```python
from build123d import *

# Parameters (mm, degrees)
SKETCH1_W                                        = 254
SKETCH1_H                                        = 25.4
BOSS_EXTRUDE1_DEPTH                              = 12.7
SKETCH2_R                                        = 5.08
F_1_2_20_THREAD_THRU_DEPTH                       = 256.582569828
SKETCH4_R                                        = 4.1021
CUT_EXTRUDE4_DEPTH                               = 256.582569828
CSK_FOR_1_4_FLAT_HEAD_MACHINE_SCREW1_D           = 6.5278
CSK_FOR_1_4_FLAT_HEAD_MACHINE_SCREW1_CSINK_D     = 12.8778
CSK_FOR_1_4_FLAT_HEAD_MACHINE_SCREW1_CSINK_ANGLE = 82
F_1_2_20_TAPPED_HOLE3_D                          = 11.50874


with BuildPart() as part:
    # Sketch1 → Boss-Extrude1 (new body)
    with BuildSketch(Plane(origin=(0, 0, 0), x_dir=(1, 0, 0), z_dir=(0, 1, 0))):
        with Locations((-127, 12.7)):
            Rectangle(SKETCH1_W, SKETCH1_H)
    extrude(amount=BOSS_EXTRUDE1_DEPTH)

    # Sketch2 → 1/2-20 thread thru (cut, through all)
    with BuildSketch(Plane(origin=(0, 12.7, 0), x_dir=(1, 0, 0), z_dir=(0, 1, 0))):
        with Locations((-127, 12.7)):
            Circle(SKETCH2_R)
    extrude(amount=-F_1_2_20_THREAD_THRU_DEPTH, mode=Mode.SUBTRACT)

    # Sketch4 → Cut-Extrude4 (cut, through all)
    with BuildSketch(Plane.XZ):
        with Locations(Location((-211.4804, -12.7, 0), (0, 0, 270))):
            Circle(SKETCH4_R)
        with Locations(Location((-42.5196, -12.7, 0), (0, 0, 270))):
            Circle(SKETCH4_R)
    extrude(amount=-CUT_EXTRUDE4_DEPTH, mode=Mode.SUBTRACT)

    # CSK for 1/4 Flat Head Machine Screw1 (through all)
    with Locations(Plane(origin=(0, 0, 0), x_dir=(-1, 0, 0), z_dir=(0, -1, 0))):
        with Locations((241.3, 12.7), (12.7, 12.7)):
            CounterSinkHole(CSK_FOR_1_4_FLAT_HEAD_MACHINE_SCREW1_D / 2, CSK_FOR_1_4_FLAT_HEAD_MACHINE_SCREW1_CSINK_D / 2, counter_sink_angle=CSK_FOR_1_4_FLAT_HEAD_MACHINE_SCREW1_CSINK_ANGLE)

    # 1/2-20 Tapped Hole3 (through all)
    with Locations(Plane(origin=(0, 12.7, 0), x_dir=(1, 0, 0), z_dir=(0, 1, 0))):
        with Locations((-127, 12.7)):
            Hole(F_1_2_20_TAPPED_HOLE3_D / 2)


solid = part.part
```
The listing builds one solid part. Answer for the finished solid, in the listing's coordinates (mm). Round coordinates to 2 decimals unless told otherwise and drop trailing zeros. Write each loop counter-clockwise with the first axis right and the second up, starting at its lowest first coordinate (ties: lowest second). Pieces come first, ordered by that corner, then holes. Notation, with made-up numbers: (46.25, 47.5) -> (60.25, 47.5) arc R30 ccw to (60.25, 86.5) -> close; hole circle Ø4 at (-28, 11). An arc over 180 degrees is marked (long way). Use CSV: the item, a comma, the result in double quotes. Start each with the question number.
(1) This flat-tipped pin is pushed along its axis until it touches: pin 1 (3 mm diameter, centred on x = -93, z = -9.5, fed in from -Y). Where does it stop, or does it pass through?
(2) Section A-A on x = -127 is taken. Give the vertices of the cut face in (y, z).
(3) Consider L1, parallel to Z at x = -127, y = 9; L2, parallel to Z at x = -12.7, y = 9; L3, parallel to X at y = 9, z = -15. Determine where each line is inside the solid, lowest interval first. Write a range as from..to.
(4) The mould has two halves that part along X. Classify faces 1 (the face through (-238.04, 3.475, -13.727)), 2 (the face through (-129, 12.7, -19)), 3 (the face through (0, 6, -13)): released by +X, released by -X, zero draft, split by the parting line, or undercut.
(5) Section D-D on x = -12.7 is taken. Give the vertices of the cut face in (y, z).
(6) Section C-C on y = 10.5 is taken. Give the vertices of the cut face in (x, z), then the cut area to 3 significant figures.
(7) Section B-B on z = -12.7 is taken. Give the vertices of the cut face in (x, y), then the cut area to 3 significant figures.
A:
1,pin 1,"stops at y = 0"
2,outline,"(0, -25.4) -> (12.7, -25.4) -> (12.7, -18.45) -> (0, -18.45) -> close; (0, -6.95) -> (12.7, -6.95) -> (12.7, 0) -> (0, 0) -> close"
3,L1,"z = -25.4..-18.45, -6.95..0"
3,L2,"z = -25.4..-15.96, -9.44..0"
3,L3,"x = -254..-243.62, -238.98..-214.88, -208.08..-132.27, -121.73..-45.92, -39.12..-15.02, -10.38..0"
4,face 1,"undercut"
4,face 2,"zero draft"
4,face 3,"released by +X"
5,outline,"(0, -25.4) -> (12.7, -25.4) -> (12.7, -15.96) -> (3.65, -15.96) -> (0, -19.14) -> close; (0, -6.26) -> (3.65, -9.44) -> (12.7, -9.44) -> (12.7, 0) -> (0, 0) -> close"
6,outline,"(-254, -25.4) -> (0, -25.4) -> (0, 0) -> (-254, 0) -> close; hole circle Ø6.53 at (-241.3, -12.7); hole circle Ø8.2 at (-211.48, -12.7); hole circle Ø11.51 at (-127, -12.7); hole circle Ø8.2 at (-42.52, -12.7); hole circle Ø6.53 at (-12.7, -12.7)"
6,area,"6,170 mm²"
7,outline,"(-254, 0) -> (-247.74, 0) -> (-244.56, 3.65) -> (-244.56, 12.7) -> (-254, 12.7) -> close; (-238.04, 3.65) -> (-234.86, 0) -> (-215.58, 0) -> (-215.58, 12.7) -> (-238.04, 12.7) -> close; (-207.38, 0) -> (-132.75, 0) -> (-132.75, 12.7) -> (-207.38, 12.7) -> close; (-121.25, 0) -> (-46.62, 0) -> (-46.62, 12.7) -> (-121.25, 12.7) -> close; (-38.42, 0) -> (-19.14, 0) -> (-15.96, 3.65) -> (-15.96, 12.7) -> (-38.42, 12.7) -> close; (-9.44, 3.65) -> (-6.26, 0) -> (0, 0) -> (0, 12.7) -> (-9.44, 12.7) -> close"
7,area,"2,680 mm²"
